Build history of the part. All positions in model axes, mm. Coordinates: 2 decimals unless noted, no trailing zeros. Order: outer loops, then holes, each group sorted by start corner. A loop starts at its lowest first (then second) coordinate and runs counter-clockwise, first axis right, second up. Notation, with made-up numbers: (-16, 49.5) - (35, 49.5) arc R21 ccw to (35, 71.5) - close; hole circle Ø2 at (57.25, 53.5). An arc over 180 degrees is marked (long way). Write each question's results on one line, items separated by ' | '.
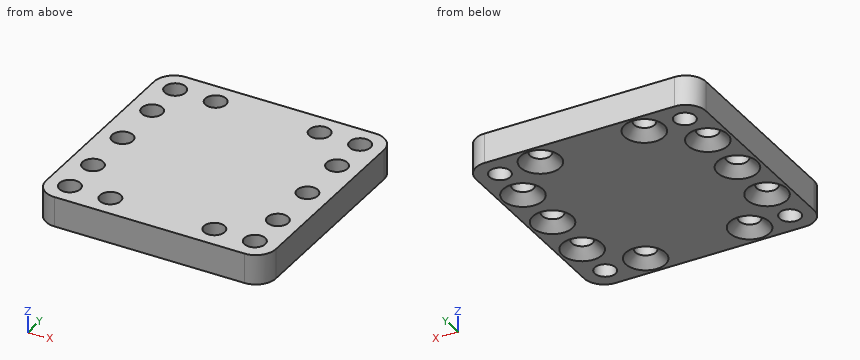
Autodesk Inventor part; units mm, degrees
ref_plane "YZ Plane" through (0, 0, 0) normal (1, 0, 0) x (0, 1, 0)
ref_plane "XZ Plane" through (0, 0, 0) normal (0, 1, 0) x (-1, 0, 0)
ref_plane "XY Plane" through (0, 0, 0) normal (0, 0, 1) x (1, 0, 0)
sketch "Sketch1" plane through (0, 0, 0) normal (0, 0, 1) x (1, 0, 0)
  line L0 (0, 51.1175) -> (0, -51.1175)
  line L1 (-51.1175, 0) -> (51.1175, 0)
  line L2 (36.5125, -36.5125) -> (-36.5125, -36.5125)
  line L3 (-36.5125, -36.5125) -> (-36.5125, 36.5125)
  line L4 (-36.5125, 36.5125) -> (36.5125, 36.5125)
  line L5 (36.5125, 36.5125) -> (36.5125, -36.5125)
  line L6 (36.5125, -36.5125) -> (-36.5125, 36.5125) construction
  line L7 (-36.5125, -36.5125) -> (36.5125, 36.5125) construction
  line L8 (29.3688, -29.3688) -> (-29.3688, -29.3688) construction
  line L9 (-29.3688, -29.3688) -> (-29.3688, 29.3687) construction
  line L10 (-29.3688, 29.3687) -> (29.3688, 29.3687) construction
  line L11 (29.3688, 29.3687) -> (29.3688, -29.3688) construction
  line L12 (29.3688, -29.3688) -> (-29.3688, 29.3687) construction
  line L13 (-29.3688, -29.3688) -> (29.3688, 29.3687) construction
  point P0 (0, 0)
  dimension "d0" = 73.025
  dimension "d1" = 58.7375
extrude "Extrusion1" add sketch "Sketch1" along normal blind 9.525
hole "Hole1" at (-29.3688, 29.3687, 0) at (29.3688, 29.3687, 0) at (29.3688, -29.3688, 0) at (-29.3688, -29.3688, 0) direction (0, 0, 1) diameter 6.647 end through all
sketch "Sketch2" plane through (0, 0, 0) normal (0, 0, -1) x (-1, 0, 0)
  line L0 (-36.5125, 36.5125) -> (36.5125, 36.5125)
  line L1 (-29.3688, 29.3687) -> (-29.3688, -29.3688) construction
  line L2 (29.3688, -29.3688) -> (29.3688, 29.3687) construction
  line L3 (29.3688, 29.3687) -> (-29.3688, 29.3687) construction
  line L4 (-29.3688, -29.3688) -> (29.3688, -29.3688) construction
  line L5 (16.5125, -29.3687) -> (-16.5125, -29.3687) construction
  line L6 (-16.5125, -29.3687) -> (-16.5125, 29.3687) construction
  line L7 (-16.5125, 29.3687) -> (16.5125, 29.3687) construction
  line L8 (16.5125, 29.3687) -> (16.5125, -29.3687) construction
  line L9 (16.5125, -29.3687) -> (-16.5125, 29.3687) construction
  line L10 (-16.5125, -29.3687) -> (16.5125, 29.3687) construction
  line L11 (-36.5125, -36.5125) -> (-36.5125, 36.5125) construction
  line L12 (29.3688, -16.5125) -> (-29.3688, -16.5125) construction
  line L13 (-29.3688, -16.5125) -> (-29.3688, 16.5125) construction
  line L14 (-29.3688, 16.5125) -> (29.3688, 16.5125) construction
  line L15 (29.3688, 16.5125) -> (29.3688, -16.5125) construction
  line L16 (29.3688, -16.5125) -> (-29.3688, 16.5125) construction
  line L17 (-29.3688, -16.5125) -> (29.3688, 16.5125) construction
  point P0 (0, 0)
  point P1 (-29.3688, 0)
  point P2 (29.3688, 0)
  point P3 (0, 29.3687)
  point P4 (0, -29.3688)
  dimension "d12" = 20
  dimension "d21" = 20
hole "Hole2" at (-16.5125, 29.3687, 0) at (16.5125, -29.3687, 0) at (29.3688, 0, 0) at (-29.3688, 0, 0) at (16.5125, 29.3687, 0) at (-16.5125, -29.3687, 0) at (29.3688, 16.5125, 0) at (29.3688, -16.5125, 0) at (-29.3688, -16.5125, 0) at (-29.3688, 16.5125, 0) direction (0, 0, 1) diameter 6.604 end through all countersink diameter 12.5984 countersink angle 90
fillet "Fillet1" radius 6.35 4 edges at (-36.5125, -36.5125, 4.7625) (-36.5125, 36.5125, 4.7625) (36.5125, -36.5125, 4.7625) (36.5125, 36.5125, 4.7625)
sketch "Sketch3" plane through (0, 0, 9.525) normal (0, 0, 1) x (1, 0, 0)
  point P0 (0, 0)
1. Probe line 1 (X direction, y = 19.5, z = 7.75); line 2 (Y direction, x = -32, z = 7) (1 decimal); line 3 (Y direction, x = -28, z = 8.75). List the from-to ranges inside material, lowest first.
Solved:
line 1: x = -36.51 to -30.78, -27.96 to 27.96, 30.78 to 36.51 | line 2: y = -36.2 to -31.4, -27.3 to -18.5, -14.5 to -2, 2 to 14.5, 18.5 to 27.3, 31.4 to 36.2 | line 3: y = -36.51 to -32.4, -26.34 to -19.52, -13.51 to -3, 3 to 13.51, 19.52 to 26.34, 32.4 to 36.51
2. Band-saw the part on B-B on z = 7.5. Give the number of separate pieces and of enclosed holes in the cut face, then the cut area to 3 significant figures.
Solved:
separate pieces: 1 | enclosed holes: 14 | area: 4,820 mm2
3. Drop a flat-ended pin along its axis: pin 1 Ø8.5 at (x, y) = (16.51, 29.37) entering from -Z. Give the stop position or say it passes through.
Solved:
pin 1: stops at z = 2.05
4. Band-saw the part on A-A on y = 0. Give the cut face in (x, z) (1 decimal).
Solved:
outline: (-36.5, 0) - (-35.7, 0) - (-32.7, 3) - (-32.7, 9.5) - (-36.5, 9.5) - close; (-26.1, 3) - (-23.1, 0) - (23.1, 0) - (26.1, 3) - (26.1, 9.5) - (-26.1, 9.5) - close; (32.7, 3) - (35.7, 0) - (36.5, 0) - (36.5, 9.5) - (32.7, 9.5) - close
